For this review, use the dimensioned drawing (mm, ordinates from the lowest corner) and the shaded views. A direction names the side the tool comes from. Give positions to 0.01 mm unless a question says otherwise; leave off trailing zeros. Loops run counter-clockwise (first coordinate to the right, second up) from the corner with the lowest first, then second, coordinate; pieces in that order, holes last. Notation, with made-up numbers: (-2, 53) - (3, 53) arc R22 cw to (3, 69) - close; hole circle Ø5 at (-17, 59). An arc over 180 degrees is marked (long way). Put each result on its own line as item: value.
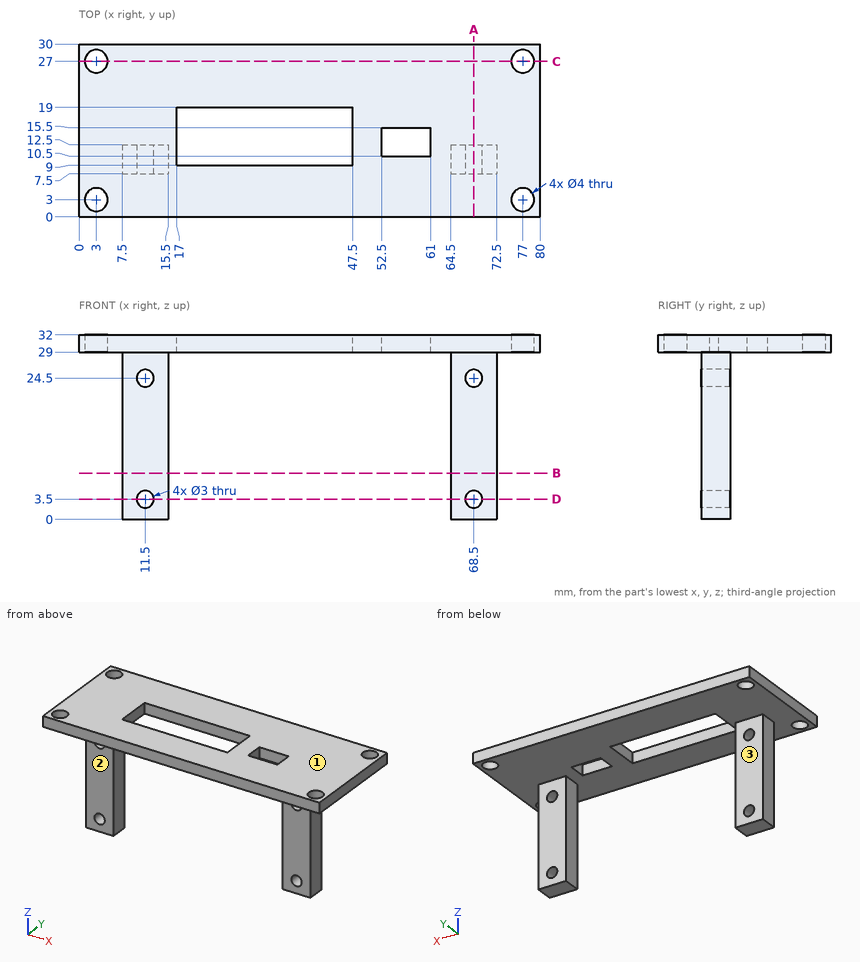
1) Wall thickness on line 1 (Y direction, x = 77, z = 31.35); line 2 (Z direction, x = 11.5, y = 11.4); line 3 (X direction, y = 9, z = 12): over which ranges is each line inside the solid? List them lowest first.
Geometry check:
line 1: y = 0 to 1, 5 to 25, 29 to 30
line 2: z = 0 to 2, 5 to 23, 26 to 32
line 3: x = 7.5 to 15.5, 64.5 to 72.5
2) Take a section at B-B on z = 8. State the section outline as (x, y) points, and give its area (3 significant figures).
Geometry check:
outline: (7.5, 7.5) - (15.5, 7.5) - (15.5, 12.5) - (7.5, 12.5) - close; (64.5, 7.5) - (72.5, 7.5) - (72.5, 12.5) - (64.5, 12.5) - close
area: 80.0 mm²
3) Take a section at D-D on z = 3.5. State the section outline as (x, y) points, and give its area (3 significant figures).
Geometry check:
outline: (7.5, 7.5) - (10, 7.5) - (10, 12.5) - (7.5, 12.5) - close; (13, 7.5) - (15.5, 7.5) - (15.5, 12.5) - (13, 12.5) - close; (64.5, 7.5) - (67, 7.5) - (67, 12.5) - (64.5, 12.5) - close; (70, 7.5) - (72.5, 7.5) - (72.5, 12.5) - (70, 12.5) - close
area: 50.0 mm²
4) Take a section at A-A on x = 68.5. State the section outline as (y, z) points.
Geometry check:
outline: (0, 29) - (7.5, 29) - (7.5, 26) - (12.5, 26) - (12.5, 29) - (30, 29) - (30, 32) - (0, 32) - close; (7.5, 0) - (12.5, 0) - (12.5, 2) - (7.5, 2) - close; (7.5, 5) - (12.5, 5) - (12.5, 23) - (7.5, 23) - close
5) For the marked faces 1, 2 and 3, list the 3-axis set-ups (+Z, -Z, +X, -X, +Y, -Y) from which the entire face can be reached by the end or side of a thin tool; tool diameter is ignored.
Geometry check:
face 1: +Z, +X, -X, +Y, -Y
face 2: -Z, +X, -X, -Y
face 3: -Z, +X, -X, +Y
6) Insertion check: pin 1 Ø6.5 at (x, z) = (68.5, 8) entering from +Y; pin 2 Ø2.5 at (y, z) = (9, 11) entering from +X; pin 3 Ø2.5 at (x, z) = (13, 12) entering from -Y. Each pin has a flat end and moves straight along its axis. Give the tip position at first contact, or say it passes through.
Geometry check:
pin 1: stops at y = 12.5
pin 2: stops at x = 72.5
pin 3: stops at y = 7.5
7) Take a section at C-C on y = 27. State the section outline as (x, z) points.
Geometry check:
outline: (0, 29) - (1, 29) - (1, 32) - (0, 32) - close; (5, 29) - (75, 29) - (75, 32) - (5, 32) - close; (79, 29) - (80, 29) - (80, 32) - (79, 32) - close
